Geometry: final body of the model. Coordinates: model frame, mm. A direction names the side the tool comes from. Round coordinates to 2 decimals unless told otherwise and drop trailing zeros. Loops run counter-clockwise (first coordinate to the right, second up) from the corner with the lowest first, then second, coordinate; pieces in that order, holes last. Notation, with made-up numbers: (88.25, -14.5) -> (125.25, -14.5) arc R18 cw to (125.25, 18.5) -> close; hole circle Ø8 at (1.25, -38.75). An arc over 180 degrees is marked (long way). Answer in a Markdown table with one row per item.
```python
from build123d import *

# Parameters (mm, degrees)
SKETCH_1_R          = 5
EXTRUDE_1_DEPTH     = 1
SKETCH_2_R          = 3.5
SKETCH_2_R_2        = 2.5
EXTRUDE_2_DEPTH     = 1
CUT_EXTRUDE_START   = -5
SKETCH_3_R          = 2.5
CUT_EXTRUDE_1_DEPTH = 5


with BuildPart() as part:
    # 草图1 → 凸台-拉伸1 (new body)
    with BuildSketch(Plane.XY):
        Circle(SKETCH_1_R)
    extrude(amount=EXTRUDE_1_DEPTH)

    # 草图2 → 凸台-拉伸2 (add)
    with BuildSketch(Plane.XY.offset(1)):
        Circle(SKETCH_2_R)
        Circle(SKETCH_2_R_2, mode=Mode.SUBTRACT)
    extrude(amount=EXTRUDE_2_DEPTH)

    # 草图3 → 切除-拉伸1 (cut)
    with BuildSketch(Plane.XY.offset(1).offset(CUT_EXTRUDE_START)):
        Circle(SKETCH_3_R)
    extrude(amount=CUT_EXTRUDE_1_DEPTH, mode=Mode.SUBTRACT)


solid = part.part
```
Item 1: Ray query, L1, parallel to Y at x = 0, z = 1.2; L2, parallel to Y at x = 0, z = 0.8; L3, parallel to Z at x = -2.5, y = 2.75. Return the intervals inside material, ascending.
Ans:
| item | result |
|---|---|
| L1 | -3.5 to -2.5, 2.5 to 3.5 |
| L2 | -5 to -2.5, 2.5 to 5 |
| L3 | 0 to 1 |
Item 2: Set-up query: faces 4 (the flat face through (2, -2, 0)), 5 (the cylindrical face through (3.233, -1.341, 1.493)). Return all of +Z, -Z, +X, -X, +Y, -Y with unobstructed straight access to the full face (end or side cutting, diameter ignored); none if empty.
Ans:
| item | result |
|---|---|
| face 4 | -Z, +X, -X, +Y, -Y |
| face 5 | +Z |
Item 3: Section query D-D, the plane y = -3. Output: boundary loops of the cut face in (x, z).
Ans:
| item | result |
|---|---|
| outline | (-4, 0) -> (4, 0) -> (4, 1) -> (1.8, 1) -> (1.8, 2) -> (-1.8, 2) -> (-1.8, 1) -> (-4, 1) -> close |
Item 4: Mould query, pull axis X, two halves, no side actions, for faces 1 (the cylindrical face through (-1.08, -4.88, 0.49)), 2 (the flat face through (2, -2, 2)), 3 (the cylindrical face through (-0.54, -2.44, 0.99)). Classes: released by +X, released by -X, zero draft, split by the parting line, or undercut.
Ans:
| item | result |
|---|---|
| face 1 | split by the parting line |
| face 2 | zero draft |
| face 3 | undercut |
Item 5: Section query A-A, the plane y = 0. Output: boundary loops of the cut face in (x, z).
Ans:
| item | result |
|---|---|
| outline | (-5, 0) -> (-2.5, 0) -> (-2.5, 2) -> (-3.5, 2) -> (-3.5, 1) -> (-5, 1) -> close; (2.5, 0) -> (5, 0) -> (5, 1) -> (3.5, 1) -> (3.5, 2) -> (2.5, 2) -> close |
Item 6: Section query C-C, the plane z = 1.2. Output: boundary loops of the cut face in (x, y).
Ans:
| item | result |
|---|---|
| outline | circle Ø7 at (0, 0); hole circle Ø5 at (0, 0) |
Item 7: First-contact query: P1, Ø6, axis at x = 3.5, y = -3, coming from the +Z side; P2, Ø4, axis at x = 0, y = 0, coming from the +Z side. Flat tips, straight axial feed; report the tip coordinate or a pass-through.
Ans:
| item | result |
|---|---|
| P1 | z = 2 |
| P2 | through |
